Geometry: final body of the model. Coordinates: model frame, mm. A direction names the side the tool comes from. Give positions to 0.01 mm unless a question says otherwise; leave off trailing zeros. Order: outer loops, then holes, each group sorted by start corner. A loop starts at its lowest first (then second) coordinate and runs counter-clockwise, first axis right, second up. Notation, with made-up numbers: (9.5, 35) -> (41.5, 35) arc R15 ccw to (41.5, 58) -> close; hole circle Ø10 at (-8.75, 41.25). An arc over 180 degrees is marked (long way). Answer in a Markdown table with one row per item. Add a question column.
Q1. Set-up query: faces 4 (the face through (-2.11, 3.49, -1.77)), 5 (the face through (-68, 2.5, -96)). Return all of +Z, -Z, +X, -X, +Y, -Y with unobstructed straight access to the full face (end or side cutting, diameter ignored); none if empty.
Q2. Cut plane A-A on z = -2.7. Return the cut outline in (x, y), and give its area (3 significant figures).
Q3. Line query: line 1 along Z through (x, y) = (-67.3, 1.05); line 2 along X through (y, z) = (1.4, -2.7); line 3 along Z through (x, y) = (-2.7, 3.05). Output: solid intervals per line, ascending. Write a range as from..to.
Q4. Pull-direction query (Z, two-part tool) for faces 1 (the face through (-65.2, 1.23, -2.04)), 2 (the face through (-35, 1, -102)), 3 (the face through (2, 1, -49)); classes: +Z half, -Z half, draft (parallel to the pull), parting line (faces both ways), or undercut.
Q5. Contact query for a flat-ended pin moving along its axis: P1, Ø2, axis at x = -3, z = -2.5, coming from the -Y side. Output: stop coordinate, or through.
Q6. Cut plane B-B on x = -2.7. Return the cut outline in (y, z), and give its area (3 significant figures).
Autodesk Inventor part; units mm, degrees
ref_plane "Work Plane3" through (2, 0, -50) normal (0, 0, -1) x (-1, 0, 0)
ref_plane "Work Plane4" through (-35, 0, -102) normal (-1, 0, 0) x (0, 0, 1)
ref_plane "YZ Plane" through (0, 0, 0) normal (1, 0, 0) x (0, 1, 0)
sketch "Sketch1" plane through (0, 0, 0) normal (0, 1, 0) x (-1, 0, 0)
  line L0 (0, 0) -> (70, 0) construction
  line L1 (70, 0) -> (70, -100) construction
  line L2 (70, -100) -> (0, -100) construction
  line L3 (0, -100) -> (0, 0) construction
  circle A0 centre (2.7, -97.3) radius 1.7 construction
  line L4 (0, -95.6) -> (4.4, -95.6) construction
  line L5 (4.4, -95.6) -> (4.4, -100) construction
  line L6 (72, 2) -> (-2, 2)
  line L7 (-2, 2) -> (-2, -102)
  line L8 (-2, -102) -> (72, -102)
  line L9 (72, -102) -> (72, 2)
  circle A1 centre (2.7, -97.3) radius 2.2
  dimension "d0" = 100
  dimension "d1" = 70
  dimension "d2" = 3.4
  dimension "d3" = 4.4
  dimension "d4" = 4.4
  dimension "d5" = 2
  dimension "d6" = 0.5
extrude "Extrusion3" add sketch "Sketch1" along normal blind 4.5 contours L9 L8 L7 L6 | A1
extrude "Extrusion4" cut sketch "Sketch1" along normal blind 2.5 contours A1
sketch "Sketch3" plane through (-2.7, 2.5, -97.3) normal (0, -1, 0) x (1, 0, 0)
  circle A0 centre (0, 0) radius 2.2
  circle A1 centre (0, 0) radius 1.1
  point P0 (2.7, 97.3)
  dimension "d16" = 2.2
extrude "Extrusion5" cut sketch "Sketch3" against normal up to surface (2 mm away) contours A1
ref_plane "Work Plane3" through (2, 0, -50) normal (0, 0, -1) x (-1, 0, 0)
ref_plane "Work Plane4" through (-35, 0, -102) normal (-1, 0, 0) x (0, 0, 1)
mirror "Mirror1" about plane through (-35, 0, -102) normal (-1, 0, 0) of "Extrusion4", "Extrusion5"
mirror "Mirror2" about plane through (2, 0, -50) normal (0, 0, -1) of "Extrusion4", "Extrusion5", "Mirror1"
chamfer "Chamfer1" distance 2 angle 45 8 edges at (-72, 2.25, 2) (2, 2.25, 2) (-72, 2.25, -102) (2, 2.25, -102) (-35, 4.5, -102) (2, 4.5, -50) (-72, 4.5, -50) (-35, 4.5, 2)
properties part number "basePlate"
Completed:
| question | item | result |
|---|---|---|
| 1 | face 4 | +Y, -Y |
| 1 | face 5 | -Y |
| 2 | outline | (-72, 0) -> (-69.5, 0) -> (-69.5, 2.5) -> (-68.4, 2.5) -> (-68.4, 4.5) -> (-70, 4.5) -> (-72, 2.5) -> close; (-66.2, 2.5) -> (-65.1, 2.5) -> (-65.1, 0) -> (-4.9, 0) -> (-4.9, 2.5) -> (-3.8, 2.5) -> (-3.8, 4.5) -> (-66.2, 4.5) -> close; (-1.6, 2.5) -> (-0.5, 2.5) -> (-0.5, 0) -> (2, 0) -> (2, 2.5) -> (0, 4.5) -> (-1.6, 4.5) -> close |
| 2 | area | 298 mm² |
| 3 | line 1 | z = -102..-99.5, -95.1..-4.9, -0.5..2 |
| 3 | line 2 | x = -72..-69.5, -65.1..-4.9, -0.5..2 |
| 3 | line 3 | z = -101.45..-98.4, -96.2..-3.8, -1.6..1.45 |
| 4 | face 1 | undercut |
| 4 | face 2 | -Z half |
| 4 | face 3 | draft |
| 5 | P1 | stops at y = 2.5 |
| 6 | outline | (0, -102) -> (2.5, -102) -> (4.5, -100) -> (4.5, -98.4) -> (2.5, -98.4) -> (2.5, -99.5) -> (0, -99.5) -> close; (0, -95.1) -> (2.5, -95.1) -> (2.5, -96.2) -> (4.5, -96.2) -> (4.5, -3.8) -> (2.5, -3.8) -> (2.5, -4.9) -> (0, -4.9) -> close; (0, -0.5) -> (2.5, -0.5) -> (2.5, -1.6) -> (4.5, -1.6) -> (4.5, 0) -> (2.5, 2) -> (0, 2) -> close |
| 6 | area | 433 mm² |
